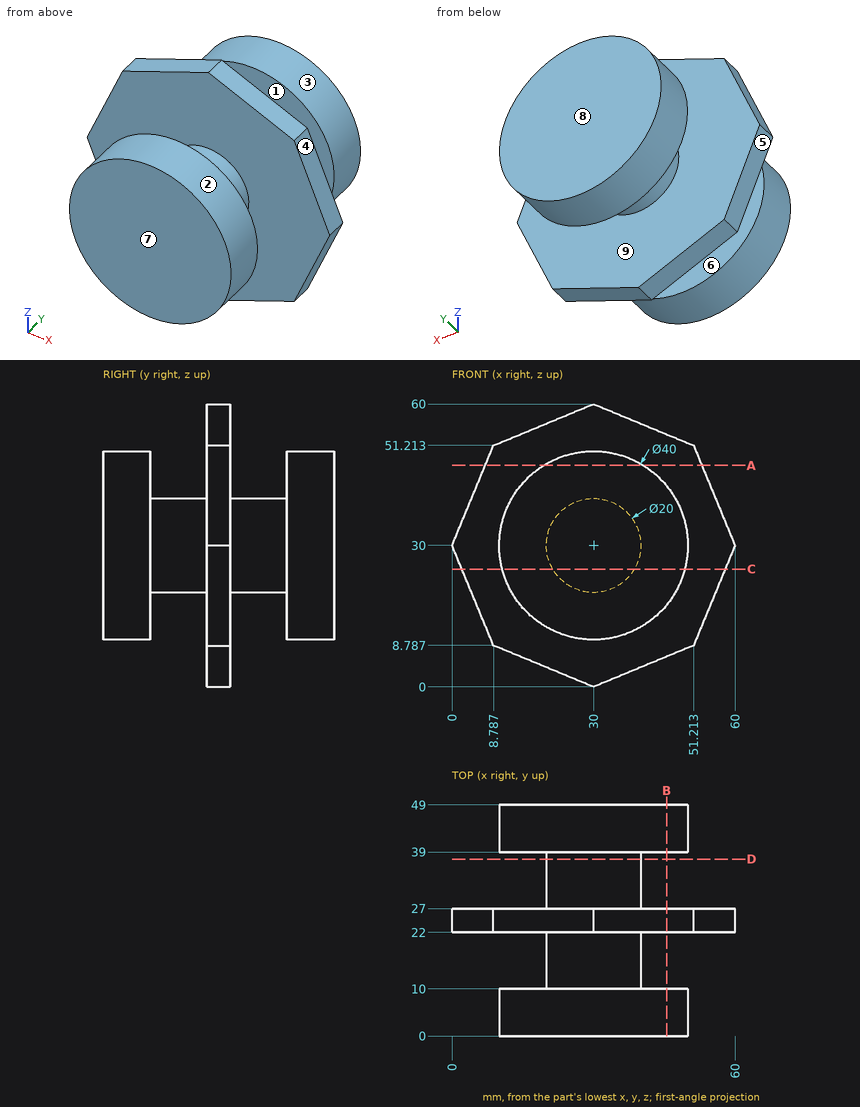
The drawing under review shows one solid part. Ordinate dimensions are in mm from its lowest x, y, z. A direction names the side the tool comes from. Round coordinates to 2 decimals unless told otherwise and drop trailing zeros. Order: outer loops, then holes, each group sorted by start corner. A loop starts at its lowest first (then second) coordinate and runs counter-clockwise, first axis right, second up. Notation, with made-up numbers: (67.5, 46.25) -> (96.5, 46.25) arc R11 ccw to (96.5, 66.25) -> close; hole circle Ø6 at (56.25, 72.25). An arc over 180 degrees is marked (long way). Return JSON: item names as keys, results as strings.
1. For the marked faces 1, 2, 3, 4 and 5, list the 3-axis set-ups (+Z, -Z, +X, -X, +Y, -Y) from which the entire face can be reached by the end or side of a thin tool; tool diameter is ignored.
Answer block:
{"face 1": "none", "face 2": "-Y", "face 3": "+Y", "face 4": "+Z, +X, +Y, -Y", "face 5": "-Z, -X, +Y, -Y"}
2. Take a section at A-A (z = 47). Write out the cut boundary in (x, y).
Answer block:
{"outline": "(7.04, 22) -> (52.96, 22) -> (52.96, 27) -> (7.04, 27) -> close; (19.46, 0) -> (40.54, 0) -> (40.54, 10) -> (19.46, 10) -> close; (19.46, 39) -> (40.54, 39) -> (40.54, 49) -> (19.46, 49) -> close"}
3. Take a section at D-D (y = 37.5). Write out the cut boundary in (x, z), then the cut area to 3 significant figures.
Answer block:
{"outline": "circle Ø20 at (30, 30)", "area": "314 mm²"}
4. Insertion check: P1, Ø1.5, axis at x = 23, z = 8, coming from the +Y side; P2, Ø1, axis at x = 45.5, z = 10.5, coming from the -Y side; P3, Ø12, axis at x = 13.5, y = 24.5, coming from the -Z side. Each pin has a flat end and moves straight along its axis. Give the tip position at first contact, or say it passes through.
Answer block:
{"P1": "stops at y = 27", "P2": "stops at y = 22", "P3": "stops at z = 4.35"}
5. Take a section at B-B (x = 45.5). Write out the cut boundary in (y, z), then the cut area to 3 significant figures.
Answer block:
{"outline": "(0, 17.36) -> (10, 17.36) -> (10, 42.64) -> (0, 42.64) -> close; (22, 6.42) -> (27, 6.42) -> (27, 53.58) -> (22, 53.58) -> close; (39, 17.36) -> (49, 17.36) -> (49, 42.64) -> (39, 42.64) -> close", "area": "741 mm²"}
6. For L1, parallel to Y at x = 38, z = 20; L2, parallel to X at y = 21.5, z = 29.5; L3, parallel to Y at x = 21.5, z = 56, list the stretches that pass through material, from the lowest coordinate up. Write a range as [from, to].
Answer block:
{"L1": "y = [0, 10], [22, 27], [39, 49]", "L2": "x = [20.01, 39.99]", "L3": "y = [22, 27]"}
7. Take a section at C-C (z = 25). Write out the cut boundary in (x, y) (1 decimal), then the cut area to 3 significant figures.
Answer block:
{"outline": "(2.1, 22) -> (21.3, 22) -> (21.3, 10) -> (10.6, 10) -> (10.6, 0) -> (49.4, 0) -> (49.4, 10) -> (38.7, 10) -> (38.7, 22) -> (57.9, 22) -> (57.9, 27) -> (38.7, 27) -> (38.7, 39) -> (49.4, 39) -> (49.4, 49) -> (10.6, 49) -> (10.6, 39) -> (21.3, 39) -> (21.3, 27) -> (2.1, 27) -> close", "area": "1,470 mm²"}
8. The part is to be moulded in two halves that separate along Y. For the marked faces 6, 7, 8 and 9, say which applies: +Y half, -Y half, draft (parallel to the pull), parting line (faces both ways), or undercut.
Answer block:
{"face 6": "undercut", "face 7": "-Y half", "face 8": "+Y half", "face 9": "undercut"}
